Work out the finished part from the listing and answer in its coordinate system (mm). A direction names the side the tool comes from. Give positions to 0.01 mm unless a question says otherwise; leave off trailing zeros. Write each loop counter-clockwise with the first axis right and the second up, starting at its lowest first coordinate (ties: lowest second). Pieces come first, ordered by that corner, then holes. Notation, with made-up numbers: (32, -6) -> (36, -6) arc R21 cw to (36, 10) -> close; hole circle Ø7 at (12, -9.5). An arc over 180 degrees is marked (long way). Write item = value, one per line. Start each with the question number.
from build123d import *

# Parameters (mm, degrees)
SKETCH1_W           = 110
SKETCH1_H           = 70
BOSS_EXTRUDE1_DEPTH = 5
SKETCH2_W           = 90
SKETCH2_H           = 10
BOSS_EXTRUDE2_DEPTH = 20
BOSS_EXTRUDE5_DEPTH = 10
SKETCH7_R           = 5
CUT_EXTRUDE2_DEPTH  = 10
SKETCH8_R           = 4
CUT_EXTRUDE3_DEPTH  = 5
SKETCH9_W           = 5
SKETCH9_H           = 40
BOSS_EXTRUDE6_DEPTH = 10
SKETCH10_W          = 90
SKETCH10_H          = 10.075231777
BOSS_EXTRUDE7_DEPTH = 10
SKETCH11_W          = 40
SKETCH11_H          = 10
CUT_EXTRUDE4_DEPTH  = 5


with BuildPart() as part:
    # Sketch1 → Boss-Extrude1 (new body)
    with BuildSketch(Plane.XY):
        with Locations((55, 35)):
            Rectangle(SKETCH1_W, SKETCH1_H)
    extrude(amount=BOSS_EXTRUDE1_DEPTH)

    # Sketch2 → Boss-Extrude2 (add)
    with BuildSketch(Plane(origin=(0, 0, 0), x_dir=(-1, 0, 0), z_dir=(0, 0, -1))):
        with Locations((-55, 65)):
            Rectangle(SKETCH2_W, SKETCH2_H)
        Polygon((-100, 70), (-110, 70), (-110, 0), (-100, 0), (-100, 10), (-100, 60), align=None)
        Polygon((0, 70), (-10, 70), (-10, 60), (-10, 10), (-10, 0), (0, 0), align=None)
        with Locations((-55, 5)):
            Rectangle(SKETCH2_W, SKETCH2_H)
    extrude(amount=BOSS_EXTRUDE2_DEPTH)

    # Sketch6 → Boss-Extrude5 (add)
    with BuildSketch(Plane(origin=(0, 0, -20), x_dir=(-1, 0, 0), z_dir=(0, 0, -1))):
        Polygon((-45, 60), (-30, 60), (-30, 65), (-10, 65), (-10, 70), (-100, 70), (-100, 65), (-85, 65), (-85, 60), (-65, 60), (-65, 65), (-45, 65), align=None)
    extrude(amount=BOSS_EXTRUDE5_DEPTH)

    # Sketch7 → Cut-Extrude2 (cut)
    with BuildSketch(Plane(origin=(0, 70, 0), x_dir=(1, 0, 0), z_dir=(0, 1, 0))):
        with Locations((36.69, 28.79)):
            Circle(SKETCH7_R)
    extrude(amount=-CUT_EXTRUDE2_DEPTH, mode=Mode.SUBTRACT)

    # Sketch8 → Cut-Extrude3 (cut)
    with BuildSketch(Plane(origin=(0, 70, 0), x_dir=(1, 0, 0), z_dir=(0, 1, 0))):
        with Locations(Location((76.88, 19.59, 0), (0, 0, 270))):
            Circle(SKETCH8_R)
    extrude(amount=-CUT_EXTRUDE3_DEPTH, mode=Mode.SUBTRACT)

    # Sketch9 → Boss-Extrude6 (add)
    with BuildSketch(Plane(origin=(0, 0, -20), x_dir=(-1, 0, 0), z_dir=(0, 0, -1))):
        with Locations((-102.5, 35)):
            Rectangle(SKETCH9_W, SKETCH9_H)
        with Locations((-7.5, 35)):
            Rectangle(SKETCH9_W, SKETCH9_H)
    extrude(amount=BOSS_EXTRUDE6_DEPTH)

    # Sketch10 → Boss-Extrude7 (add)
    with BuildSketch(Plane(origin=(0, 0, -20), x_dir=(-1, 0, 0), z_dir=(0, 0, -1))):
        with Locations((-55, 4.962384111)):
            Rectangle(SKETCH10_W, SKETCH10_H)
    extrude(amount=BOSS_EXTRUDE7_DEPTH)

    # Sketch11 → Cut-Extrude4 (cut)
    with BuildSketch(Plane(origin=(0, 10, 0), x_dir=(1, 0, 0), z_dir=(0, 1, 0))):
        with Locations((55, 25)):
            Rectangle(SKETCH11_W, SKETCH11_H)
    extrude(amount=-CUT_EXTRUDE4_DEPTH, mode=Mode.SUBTRACT)


solid = part.part
(1) A cutting plane is placed at C-C, the plane y = 58. Write down the section's boundary in (x, z), then the cut area to 3 significant figures.
(2) Each of these flat-tipped pins is pushed along its axis until it touches: pin 1 (4 mm diameter, centred on x = 7.5, z = -25.5, fed in from +Y); pin 2 (2.5 mm diameter, centred on y = 66.5, z = -24.5, fed in from -X); pin 3 (4 mm diameter, centred on y = 62, z = -25, fed in from -X). Where does it stop, or does it pass through?
(3) Determine the mould class of faces 5 (the flat face through (85, 63, -25)), 6 (the flat face through (10, 5, -25)), 7 (the flat face through (103, 55, -25)), 8 (the flat face through (65, 62, -25)) for opening direction Y: pulls with the +Y half, pulls with the -Y half, needs draft (parallel to the pull), parting line crosses it, or undercut.
(4) A cutting plane is placed at D-D, the plane x = 76.88. Write down the section's boundary in (y, z), then the cut area to 3 significant figures.
(5) Find the intervals of material crossed by line 1 along Y through (x, z) = (60, -6); line 2 along X through (y, z) = (48, -21); line 3 along X through (y, z) = (38.5, -13), in increasing order.
(6) A cutting plane is placed at B-B, the plane x = 36.69. Write down the section's boundary in (y, z), then the cut area to 3 significant figures.
(7) A cutting plane is placed at A-A, the plane z = -28.79. State how many separate pieces and enclosed holes the cut face has, then the cut area to 3 significant figures.
(8) For faces 1 (the flat face through (100, 5, -25)), 2 (the flat face through (56, 60, -11)), 3 (the flat face through (93, 65, -25)), 4 (the flat face through (105, 35, -25)), determine the directions among +Z, -Z, +X, -X, +Y, -Y from which every point of the face is accessible in a straight line to the end or side of a thin tool.
Results list:
q1.outline = (0, -20) -> (10, -20) -> (10, 0) -> (100, 0) -> (100, -20) -> (110, -20) -> (110, 5) -> (0, 5) -> close
q1.area = 950 mm²
q2.pin_1 = 55
q2.pin_2 = 10
q2.pin_3 = 30
q3.face_5 = undercut
q3.face_6 = needs draft
q3.face_7 = pulls with the +Y half
q3.face_8 = undercut
q4.outline = (-0.08, -30) -> (10, -30) -> (10, 0) -> (60, 0) -> (60, -30) -> (70, -30) -> (70, -23.59) -> (65, -23.59) -> (65, -15.59) -> (70, -15.59) -> (70, 5) -> (0, 5) -> (0, -20) -> (-0.08, -20) -> close
q4.area = 911 mm²
q5.line_1 = 0 to 10, 60 to 70
q5.line_2 = 5 to 10, 100 to 105
q5.line_3 = 0 to 10, 100 to 110
q6.outline = (-0.08, -30) -> (5, -30) -> (5, -20) -> (10, -20) -> (10, 0) -> (60, 0) -> (60, -23.79) -> (70, -23.79) -> (70, 5) -> (0, 5) -> (0, -20) -> (-0.08, -20) -> close
q6.area = 839 mm²
q7.separate_pieces = 5
q7.enclosed_holes = 0
q7.area = 1,630 mm²
q8.face_1 = -Z, +X, -Y
q8.face_2 = -Z
q8.face_3 = -Z, +X
q8.face_4 = -Z, +X, +Y, -Y
